```python
from build123d import *

# Parameters (mm, degrees)
F0_R     = 6.35
F1_DEPTH = 25.4
F3_DEPTH = 25.401


with BuildPart() as f1:
    # F0 (on Front) → F1 (new body)
    with BuildSketch(Plane.XZ):
        with BuildLine():
            Line((-37.580457, 71.118474), (-48.764932, 14.234516))
            ThreePointArc((-48.764932, 14.234516), (0, -50.8), (48.764932, 14.234516))
            Line((48.764932, 14.234516), (69.638334, 65.191805))
            Line((69.638334, 65.191805), (21.407981, 46.068844))
            ThreePointArc((21.407981, 46.068844), (4.218409, 50.62455), (-13.488094, 48.97664))
            Line((-13.488094, 48.97664), (-37.580457, 71.118474))
        make_face()
        with Locations((-24.096556, 11.43)):
            Circle(F0_R, mode=Mode.SUBTRACT)
        with Locations((24.096556, 11.43)):
            Circle(F0_R, mode=Mode.SUBTRACT)
    extrude(amount=F1_DEPTH)

    # F2 (on face) → F3 (cut, through all)
    with BuildSketch(Plane.XZ.offset(25.4)):
        Polygon((12.603787, 8.888469), (-12.796213, 8.888469), (0, 0), align=None)
    extrude(amount=-F3_DEPTH, mode=Mode.SUBTRACT)


solid = f1.part
```
Geometry check sheet. Reference: the model listing, model coordinates, mm. A direction names the side the tool comes from. Coordinates: 2 decimals unless noted, no trailing zeros. Write each loop counter-clockwise with the first axis right and the second up, starting at its lowest first coordinate (ties: lowest second). Pieces come first, ordered by that corner, then holes. Notation, with made-up numbers: M 4.25,52.25 L 21.25,52.25 A9 cw 21.25,56.25 Z; hole C 17.5,52 d1. An arc over 180 degrees is marked long. Answer as a JSON object with one key per item and string values.
1. Go/stop test with flat-tipped pins: pin 1 Ø4 at (x, y) = (30.5, -12.5) entering from -Z; pin 2 Ø1.5 at (x, y) = (-14, -22.5) entering from +Z; pin 3 Ø2 at (x, y) = (20.5, -4) entering from +Z; pin 4 Ø7.5 at (x, z) = (-24.1, 11.43) entering from -Y. Record where each tip stops, or that it passes through.
Answers below:
{"pin 1": "stops at z = -42.05", "pin 2": "stops at z = 50.14", "pin 3": "stops at z = 46.91", "pin 4": "passes through"}
2. Tool access check on faces 1 (the flat face through (45.861, -12.522, 55.764)), 2 (the flat face through (9, 0, 11)), 3 (the flat face through (-6.49, -12.88, 4.51)). Record the directions out of +Z, -Z, +X, -X, +Y, -Y that give a thin tool (end or side, any length) a straight path to the whole face; none if there is none.
Answers below:
{"face 1": "+Z, +Y, -Y", "face 2": "+Z, -Z, +X, -X, +Y", "face 3": "+Y, -Y"}
3. Section check A-A, the plane z = 11.43. Enter the section's corners in (x, y).
Answers below:
{"outline": "M -49.5,-25.4 L -30.45,-25.4 L -30.45,0 L -49.5,0 Z; M -17.75,-25.4 L 17.75,-25.4 L 17.75,0 L -17.75,0 Z; M 30.45,-25.4 L 49.5,-25.4 L 49.5,0 L 30.45,0 Z"}
4. Scan lines: L1, parallel to X at y = -6.75, z = 16; L2, parallel to X at y = -8.5, z = 10; L3, parallel to Z at x = 8, y = -8. Record each from-to range of solid material in increasing order.
Answers below:
{"L1": "x = -48.42 to -28.51, -19.69 to 19.69, 28.51 to 49.49", "L2": "x = -49.81 to -30.28, -17.91 to 17.91, 30.28 to 49.81", "L3": "z = -50.17 to 5.64, 8.89 to 50.17"}
5. Section check D-D, the plane z = 54.5. Enter the section's corners in (x, y).
Answers below:
{"outline": "M -40.85,-25.4 L -19.5,-25.4 L -19.5,0 L -40.85,0 Z; M 42.67,-25.4 L 65.26,-25.4 L 65.26,0 L 42.67,0 Z"}
6. Draft check along X on faces 4 (the flat face through (0, -13, 8.888)), 5 (the flat face through (-43.094, -12.522, 43.075)), 6 (the flat face through (9, -25.4, 11)), 7 (the cylindrical face through (-1.319, -12.522, -50.783)). Enter one of: released by +X, released by -X, zero draft, split by the parting line, or undercut.
Answers below:
{"face 4": "undercut", "face 5": "released by -X", "face 6": "zero draft", "face 7": "split by the parting line"}
7. Section check B-B, the plane y = -3. Enter the section's corners in (x, z).
Answers below:
{"outline": "M -48.76,14.23 A50.8 ccw long 48.76,14.23 L 69.64,65.19 L 21.41,46.07 A50.8 ccw -13.49,48.98 L -37.58,71.12 Z; hole C -24.1,11.43 d12.7; hole M -12.8,8.89 L 0,0 L 12.6,8.89 Z; hole C 24.1,11.43 d12.7"}
8. Section check C-C, the plane x = 5. Enter the section's corners in (y, z).
Answers below:
{"outline": "M -25.4,-50.55 L 0,-50.55 L 0,3.53 L -25.4,3.53 Z; M -25.4,8.89 L 0,8.89 L 0,50.55 L -25.4,50.55 Z"}
